Can you work these out from the model? Positions are in its coordinate system, mm. Face numbers are marked on the shaded views. A direction names the side the tool comes from. Coordinates: 2 decimals unless noted, no trailing zeros. Write each loop counter-clockwise with the first axis right and the second up, starting at its lowest first coordinate (ties: lowest second). Pieces come first, ordered by that corner, then holes. Notation, with made-up numbers: (-33, 49) -> (-24, 49) arc R22 cw to (-24, 81) -> close; hole circle Ø8 at (21.5, 32.25). An arc over 180 degrees is marked (long way). Use one line per item in the form item = value.
Autodesk Fusion 360 part; units mm, degrees
sketch "Sketch1" plane through (0, 0, 0) normal (0, 0, 1) x (1, 0, 0)
  line L0 (0, 0) -> (26, 0)
  line L1 (26, 0) -> (26, 26)
  line L2 (26, 26) -> (0, 26)
  line L3 (0, 26) -> (0, 0)
  dimension "d1" = 26
  dimension "d2" = 26
extrude "Extrude1" add sketch "Sketch1" along normal blind 1
sketch "Sketch2" plane through (0, 0, 1) normal (0, 0, 1) x (-1, 0, 0)
  line L0 (0, -26) -> (0, 0)
  line L1 (0, 0) -> (-26, 0)
  line L2 (-26, 0) -> (-26, -26)
  line L3 (-26, -26) -> (0, -26)
  circle A0 centre (-23.5, -23.5) radius 1.5
  circle A1 centre (-2.5, -23.5) radius 1.5
  dimension "d5" = 3
  dimension "d6" = 3
  dimension "d7" = 2.5
  dimension "d8" = 2.5
  dimension "d9" = 2.5
  dimension "d10" = 2.5
extrude "Extrude2" cut sketch "Sketch2" against normal blind 4 contours A0 | A1
sketch "Sketch3" plane through (0, 0, 1) normal (0, 0, 1) x (-1, 0, 0)
  circle A0 centre (-2.5, -23.5) radius 1.5
  circle A1 centre (-23.5, -23.5) radius 1.5
  line L0 (0, -26) -> (0, 0)
  line L1 (0, 0) -> (-26, 0)
  line L2 (-26, 0) -> (-26, -26)
  line L3 (-26, -26) -> (0, -26)
  line L4 (-1, -16.5) -> (-5, -16.5)
  line L5 (-5, -16.5) -> (-5, -9.5)
  line L6 (-5, -9.5) -> (-1, -9.5)
  line L7 (-1, -9.5) -> (-1, -16.5)
  dimension "d13" = 7
  dimension "d14" = 4
  dimension "d15" = 1
extrude "Extrude3" add sketch "Sketch3" along normal blind 3 contours L4 L5 L6 L7
sketch "Sketch4" plane through (0, 0, 1) normal (0, 0, 1) x (-1, 0, 0)
  line L0 (-1, -9.5) -> (-1, -16.5)
  line L1 (-1, -16.5) -> (-5, -16.5)
  line L2 (-5, -16.5) -> (-5, -9.5)
  line L3 (-5, -9.5) -> (-1, -9.5)
  circle A0 centre (-2.5, -23.5) radius 1.5
  circle A1 centre (-23.5, -23.5) radius 1.5
  line L4 (0, -26) -> (0, 0)
  line L5 (0, 0) -> (-26, 0)
  line L6 (-26, 0) -> (-26, -26)
  line L7 (-26, -26) -> (0, -26)
  circle A2 centre (-22.5, -12) radius 2.5
  dimension "d19" = 5
  dimension "d20" = 3.5
extrude "Extrude4" add sketch "Sketch4" along normal blind 1 contours A2
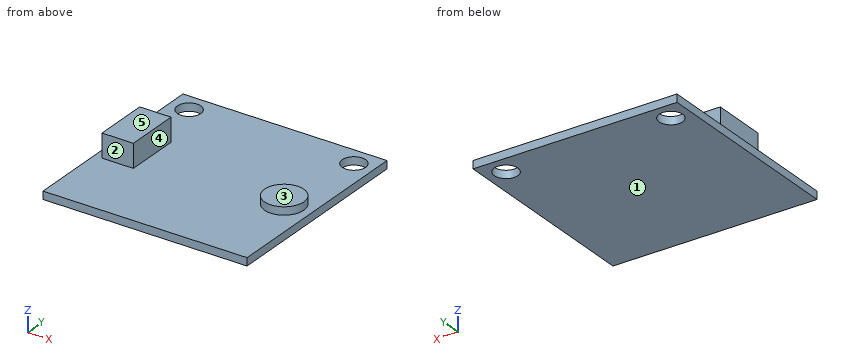
Q1. For the marked faces 1, 2 and 3, which set-ups out of +Z, -Z, +X, -X, +Y, -Y let a thin tool reach every point of the face, with its end or its side?
Return value:
face_1 = -Z, +X, -X, +Y, -Y
face_2 = +Z, +X, -X, -Y
face_3 = +Z, +X, +Y, -Y
Q2. Will these pins go through, and if not, where does the flat tip stop? pin 1 (12 mm diameter, centred on x = 10.5, y = 21.5, fed in from +Z); pin 2 (13 mm diameter, centred on x = 16.5, y = 18.5, fed in from +Z); pin 3 (1.5 mm diameter, centred on y = 12, z = 3, fed in from -X).
Return value:
pin_1 = 1
pin_2 = 2
pin_3 = 1
Q3. Thinking about a two-plate mould opening in X: for the marked faces 4 and 5, which applies, released by +X, released by -X, zero draft, split by the parting line, or undercut?
Return value:
face_4 = undercut
face_5 = zero draft
Q4. Suppose I cut it at C-C (z = 1.35). Write out the boundary of the cut face in (x, y).
Return value:
outline = (1, 9.5) -> (5, 9.5) -> (5, 16.5) -> (1, 16.5) -> close; circle Ø5 at (22.5, 12)
Q5. If I drill on line 1 (X direction, y = 23.5, z = 0.45); line 2 (Y direction, x = 2.5, z = 0.6); line 3 (Z direction, x = 2.5, y = 16.75), over which ranges is the centre line in solid material (lowest first)? Write a range as from..to.
Return value:
line_1 = 0..1, 4..22, 25..26
line_2 = 0..22, 25..26
line_3 = 0..1
Q6. Suppose I cut it at A-A (x = 2.5). Write out the boundary of the cut face in (y, z).
Return value:
outline = (0, 0) -> (22, 0) -> (22, 1) -> (16.5, 1) -> (16.5, 4) -> (9.5, 4) -> (9.5, 1) -> (0, 1) -> close; (25, 0) -> (26, 0) -> (26, 1) -> (25, 1) -> close
Q7. Suppose I cut it at D-D (y = 14). Write out the boundary of the cut face in (x, z).
Return value:
outline = (0, 0) -> (26, 0) -> (26, 1) -> (24, 1) -> (24, 2) -> (21, 2) -> (21, 1) -> (5, 1) -> (5, 4) -> (1, 4) -> (1, 1) -> (0, 1) -> close
Q8. Suppose I cut it at B-B (y = 23.5). Write out the boundary of the cut face in (x, z).
Return value:
outline = (0, 0) -> (1, 0) -> (1, 1) -> (0, 1) -> close; (4, 0) -> (22, 0) -> (22, 1) -> (4, 1) -> close; (25, 0) -> (26, 0) -> (26, 1) -> (25, 1) -> close
